Autodesk Inventor part; units mm, degrees
ref_plane "YZ Plane" through (0, 0, 0) normal (1, 0, 0) x (0, 1, 0)
ref_plane "XZ Plane" through (0, 0, 0) normal (0, 1, 0) x (-1, 0, 0)
ref_plane "XY Plane" through (0, 0, 0) normal (0, 0, 1) x (1, 0, 0)
sketch "Sketch1" plane through (0, 0, 0) normal (0, 0, 1) x (1, 0, 0)
  line L0 (0, 0) -> (23, 0) construction
  line L1 (23, 0) -> (23, 6) construction
  line L2 (23, 6) -> (0, 6) construction
  line L3 (0, 6) -> (0, 0) construction
  line L4 (0, 3) -> (23, 3) construction
  line L5 (11.5, 0) -> (11.5, 3) construction
  line L6 (11.5, 3) -> (11.5, 6) construction
  line L7 (11.5, 1.5) -> (0, 1.5) construction
  line L8 (11.5, 4.5) -> (23, 4.5) construction
  line L9 (0, 1.5) -> (11.5, 1.5) construction
  line L10 (1.5, 3) -> (10, 3)
  line L11 (10, 0) -> (1.5, 0)
  arc A0 (1.5, 3) -> (1.5, 0) centre (1.5, 1.5) ccw
  arc A1 (10, 0) -> (10, 3) centre (10, 1.5) ccw
  line L12 (11.5, 4.5) -> (23, 4.5) construction
  line L13 (13, 6) -> (21.5, 6)
  line L14 (21.5, 3) -> (13, 3)
  arc A2 (13, 6) -> (13, 3) centre (13, 4.5) ccw
  arc A3 (21.5, 3) -> (21.5, 6) centre (21.5, 4.5) ccw
  line L15 (10, 1.5) -> (13, 4.5) construction
  line L16 (11.0607, 0.4393) -> (14.0607, 3.4393)
  line L17 (11.9393, 5.5607) -> (8.9393, 2.5607)
  arc A4 (8.9393, 2.5607) -> (11.0607, 0.4393) centre (10, 1.5) ccw
  arc A5 (14.0607, 3.4393) -> (11.9393, 5.5607) centre (13, 4.5) ccw
  point P0 (5.75, 1.5)
  point P1 (17.25, 4.5)
  point P2 (11.5, 3)
  point P3 (9.3787, 3)
  point P4 (13.6213, 3)
  dimension "d6" = 23
  dimension "d7" = 6
  dimension "d8" = 3
extrude "Extrusion1" add sketch "Sketch1" along normal blind 210
properties part number "Door Seal" material "Rubber"
Could you check a few things on this model? Use its own coordinates, in mm. A direction names the side the tool comes from. Give positions to 0.01 mm unless a question says otherwise; leave off trailing zeros. Order: outer loops, then holes, each group sorted by start corner. A loop starts at its lowest first (then second) coordinate and runs counter-clockwise, first axis right, second up.
1. Suppose I cut it at B-B (x = 3.5). Write out the boundary of the cut face in (y, z).
Answers below:
outline: (0, 0) - (3, 0) - (3, 210) - (0, 210) - close
2. I need wall thicknesses on L1, parallel to Y at x = 1.5, z = 52; L2, parallel to Y at x = 14.5, z = 50; L3, parallel to X at y = 1, z = 141.5. Which ranges of each line are inside material? Lowest first, please.
Answers below:
L1: y = 0 to 3
L2: y = 3 to 6
L3: x = 0.09 to 11.62
3. Suppose I cut it at C-C (y = 1.5). Write out the boundary of the cut face in (x, z), plus the area to 3 significant figures.
Answers below:
outline: (0, 0) - (12.12, 0) - (12.12, 210) - (0, 210) - close
area: 2,550 mm2
4. Which directions (+Z, -Z, +X, -X, +Y, -Y) give clear straight access to the entire face, cutting with the end or side of a thin tool? Please do faces 1 (the flat face through (5, 3, 104)), 2 (the flat face through (18, 3, 104)), 3 (the flat face through (6, 0, 104)).
Answers below:
face 1: +Z, -Z, -X, +Y
face 2: +Z, -Z, +X, -Y
face 3: +Z, -Z, +X, -X, -Y
5. Suppose I cut it at A-A (z = 197.5). Write out the boundary of the cut face in (x, y).
Answers below:
outline: (1.5, 0) - (10, 0) arc R1.5 ccw to (11.06, 0.44) - (13.62, 3) - (21.5, 3) arc R1.5 ccw to (21.5, 6) - (13, 6) arc R1.5 ccw to (11.94, 5.56) - (9.38, 3) - (1.5, 3) arc R1.5 ccw to start
6. For pin 1 (8.5 mm diameter, centred on x = 19, z = 119.5, fed in from -Y); pin 2 (4 mm diameter, centred on x = 7, z = 102, fed in from +Y); pin 3 (4 mm diameter, centred on x = 9, z = 91.5, fed in from +Y), each with a flat end and sliding along its axis, tell me the tip position at first contact or that it passes through.
Answers below:
pin 1: stops at y = 3
pin 2: stops at y = 3
pin 3: stops at y = 4.62
